```python
from build123d import *

# Parameters (mm, degrees)
SKETCH2_R           = 12.7
SKETCH2_W           = 12.7
SKETCH2_H           = 12.7
BOSS_EXTRUDE1_DEPTH = 50.8
SKETCH3_W           = 50.8
SKETCH3_H           = 25.4
BOSS_EXTRUDE2_DEPTH = 101.6


with BuildPart() as part:
    # Sketch2 → Boss-Extrude1 (new body)
    with BuildSketch(Plane.XY):
        with BuildLine():
            Line((50.8, 25.4), (50.8, 76.2))
            ThreePointArc((50.8, 76.2), (25.4, 101.6), (0, 76.2))
            Line((0, 76.2), (0, 25.4))
            Line((0, 25.4), (0, 0))
            Line((0, 0), (50.8, 0))
            Line((50.8, 0), (50.8, 25.4))
        make_face()
        with Locations((25.4, 76.2)):
            Circle(SKETCH2_R, mode=Mode.SUBTRACT)
        with Locations((25.4, 38.1)):
            Rectangle(SKETCH2_W, SKETCH2_H, mode=Mode.SUBTRACT)
    extrude(amount=BOSS_EXTRUDE1_DEPTH)

    # Sketch3 → Boss-Extrude2 (add)
    with BuildSketch(Plane.XY):
        with Locations((25.4, 12.7)):
            Rectangle(SKETCH3_W, SKETCH3_H)
    extrude(amount=BOSS_EXTRUDE2_DEPTH)


solid = part.part
```
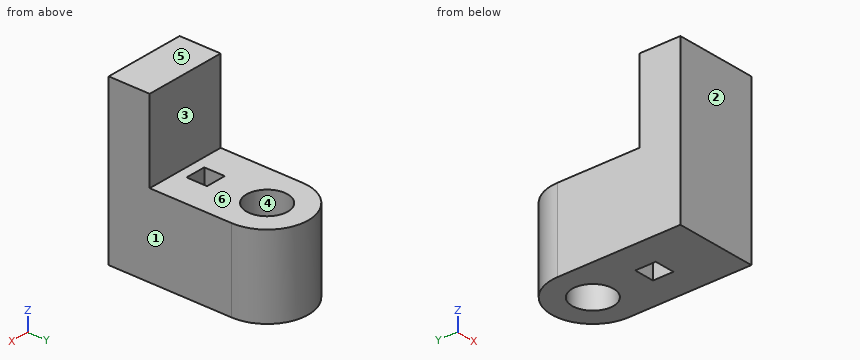
Build history of the part. All positions in model axes, mm. Face numbers are marked on the shaded views. A direction names the side the tool comes from. Give positions to 0.01 mm unless a question says otherwise; leave off trailing zeros. Order: outer loops, then holes, each group sorted by start corner. A loop starts at its lowest first (then second) coordinate and runs counter-clockwise, first axis right, second up. Notation, with made-up numbers: M -32.75,26 L 12.25,26 A24 cw 12.25,40 Z; hole C 6,-31 d9. An arc over 180 degrees is marked long. Return JSON: item names as keys, results as strings.
Q1. Band-saw the part on C-C (y = 65). Give the cut face in (x, z), then the cut area to 3 significant figures.
Answer list:
{"outline": "M 0,0 L 19.41,0 L 19.41,50.8 L 0,50.8 Z; M 31.39,0 L 50.8,0 L 50.8,50.8 L 31.39,50.8 Z", "area": "1,970 mm^2"}
Q2. Band-saw the part on A-A (x = 25.4). Give the cut face in (y, z).
Answer list:
{"outline": "M 0,0 L 31.75,0 L 31.75,50.8 L 25.4,50.8 L 25.4,101.6 L 0,101.6 Z; M 44.45,0 L 63.5,0 L 63.5,50.8 L 44.45,50.8 Z; M 88.9,0 L 101.6,0 L 101.6,50.8 L 88.9,50.8 Z"}
Q3. Wall check: probe 1 along Y at (x, z) = (25.4, 31); probe 2 along Y at (x, z) = (23.5, 41.5); probe 3 along X at (y, z) = (38, 10.5). Give the ranges that are in metal, low to high. Write a range as from..to.
Answer list:
{"probe 1": "y = 0..31.75, 44.45..63.5, 88.9..101.6", "probe 2": "y = 0..31.75, 44.45..63.64, 88.76..101.53", "probe 3": "x = 0..19.05, 31.75..50.8"}
Q4. Band-saw the part on B-B (z = 17). Give the cut face in (x, y).
Answer list:
{"outline": "M 0,0 L 50.8,0 L 50.8,76.2 A25.4 ccw 0,76.2 Z; hole C 25.4,76.2 d25.4; hole M 19.05,31.75 L 31.75,31.75 L 31.75,44.45 L 19.05,44.45 Z"}
Q5. Two-plate mould, pull along Y, no slides. Class the marked faces 1, 2, 3 and 4: pulls with the +Y half, pulls with the -Y half, needs draft (parallel to the pull), parting line crosses it, or undercut.
Answer list:
{"face 1": "needs draft", "face 2": "pulls with the -Y half", "face 3": "pulls with the +Y half", "face 4": "undercut"}
Q6. Flat gauge pins, fed straight in: pin 1 (14 mm diameter, centred on x = 27, z = 34.5, fed in from +Y); pin 2 (3 mm diameter, centred on x = 12.5, z = 23.5, fed in from +Y); pin 3 (8 mm diameter, centred on x = 11.5, y = 83.5, fed in from +Z). Where does each tip first touch, or does it go through?
Answer list:
{"pin 1": "stops at y = 101.6", "pin 2": "stops at y = 98.9", "pin 3": "stops at z = 50.8"}
Q7. 3-axis set-ups, long thin cutter, end or side, ignore diameter. For the marked faces 5 and 6: which of +Z, -Z, +X, -X, +Y, -Y reach the whole face in a straight line?
Answer list:
{"face 5": "+Z, +X, -X, +Y, -Y", "face 6": "+Z, +X, -X, +Y"}
Q8. Band-saw the part on D-D (y = 83). Give the cut face in (x, z), then the cut area to 3 significant figures.
Answer list:
{"outline": "M 0.93,0 L 14.67,0 L 14.67,50.8 L 0.93,50.8 Z; M 36.13,0 L 49.87,0 L 49.87,50.8 L 36.13,50.8 Z", "area": "1,400 mm^2"}
